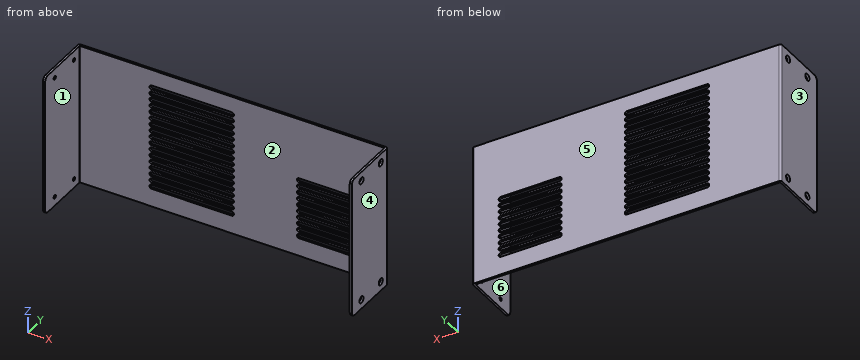
```python
from build123d import *

# Parameters (mm, degrees)
BOSS_EXTRUDE1_DEPTH                             = 132
CSK_FOR_M3_FLAT_HEAD_MACHINE_SCREW1_D           = 3.4
CSK_FOR_M3_FLAT_HEAD_MACHINE_SCREW1_DEPTH       = 5
CSK_FOR_M3_FLAT_HEAD_MACHINE_SCREW1_CSINK_D     = 6.3
CSK_FOR_M3_FLAT_HEAD_MACHINE_SCREW1_CSINK_ANGLE = 90
CSK_FOR_M3_FLAT_HEAD_MACHINE_SCREW1_TIP         = 1.021463052
CSK_FOR_M3_FLAT_HEAD_MACHINE_SCREW2_D           = 3.4
CSK_FOR_M3_FLAT_HEAD_MACHINE_SCREW2_DEPTH       = 5
CSK_FOR_M3_FLAT_HEAD_MACHINE_SCREW2_CSINK_D     = 6.3
CSK_FOR_M3_FLAT_HEAD_MACHINE_SCREW2_CSINK_ANGLE = 90
CSK_FOR_M3_FLAT_HEAD_MACHINE_SCREW2_TIP         = 1.021463052
CUT_EXTRUDE1_DEPTH                              = 5
LPATTERN1_COUNT                                 = 17
LPATTERN1_PITCH                                 = 6
CUT_EXTRUDE2_DEPTH                              = 200
LPATTERN2_COUNT                                 = 10
LPATTERN2_PITCH                                 = 6
FILLET1_R                                       = 4


with BuildPart() as part:
    # Sketch1 → Boss-Extrude1 (new body)
    with BuildSketch(Plane.XY):
        with BuildLine():
            Line((0, 0), (-2, 0))
            Line((-2, 0), (-2, 54.2))
            ThreePointArc((-2, 54.2), (-1.472792206, 55.472792206), (-0.2, 56))
            Line((-0.2, 56), (285.2, 56))
            ThreePointArc((285.2, 56), (286.472792206, 55.472792206), (287, 54.2))
            Line((287, 54.2), (287, 0))
            Line((287, 0), (285, 0))
            Line((285, 0), (285, 53.5))
            ThreePointArc((285, 53.5), (284.853553391, 53.853553391), (284.5, 54))
            Line((284.5, 54), (0.5, 54))
            ThreePointArc((0.5, 54), (0.146446609, 53.853553391), (0, 53.5))
            Line((0, 53.5), (0, 0))
        make_face()
    extrude(amount=BOSS_EXTRUDE1_DEPTH)

    # CSK for M3 Flat Head Machine Screw1
    with Locations(Plane.ZY.offset(2)):
        with Locations((8.5, 45), (8.5, 15), (123.5, 45), (123.5, 15)):
            CounterSinkHole(CSK_FOR_M3_FLAT_HEAD_MACHINE_SCREW1_D / 2, CSK_FOR_M3_FLAT_HEAD_MACHINE_SCREW1_CSINK_D / 2, depth=CSK_FOR_M3_FLAT_HEAD_MACHINE_SCREW1_DEPTH, counter_sink_angle=CSK_FOR_M3_FLAT_HEAD_MACHINE_SCREW1_CSINK_ANGLE)
            with Locations((0, 0, -(CSK_FOR_M3_FLAT_HEAD_MACHINE_SCREW1_DEPTH + CSK_FOR_M3_FLAT_HEAD_MACHINE_SCREW1_TIP / 2))):  # 118° drill point
                Cone(0, CSK_FOR_M3_FLAT_HEAD_MACHINE_SCREW1_D / 2, CSK_FOR_M3_FLAT_HEAD_MACHINE_SCREW1_TIP, mode=Mode.SUBTRACT)

    # CSK for M3 Flat Head Machine Screw2
    with Locations(Plane(origin=(287, 0, 0), x_dir=(0, 0, -1), z_dir=(1, 0, 0))):
        with Locations((-123.5, 45), (-123.5, 15), (-8.5, 45), (-8.5, 15)):
            CounterSinkHole(CSK_FOR_M3_FLAT_HEAD_MACHINE_SCREW2_D / 2, CSK_FOR_M3_FLAT_HEAD_MACHINE_SCREW2_CSINK_D / 2, depth=CSK_FOR_M3_FLAT_HEAD_MACHINE_SCREW2_DEPTH, counter_sink_angle=CSK_FOR_M3_FLAT_HEAD_MACHINE_SCREW2_CSINK_ANGLE)
            with Locations((0, 0, -(CSK_FOR_M3_FLAT_HEAD_MACHINE_SCREW2_DEPTH + CSK_FOR_M3_FLAT_HEAD_MACHINE_SCREW2_TIP / 2))):  # 118° drill point
                Cone(0, CSK_FOR_M3_FLAT_HEAD_MACHINE_SCREW2_D / 2, CSK_FOR_M3_FLAT_HEAD_MACHINE_SCREW2_TIP, mode=Mode.SUBTRACT)

    # Sketch6 → Cut-Extrude1 (cut)
    with BuildSketch(Plane(origin=(0, 56, 0), x_dir=(1, 0, 0), z_dir=(0, 1, 0))):
        with BuildLine():
            Line((67.2, -17), (142.2, -17))
            ThreePointArc((142.2, -17), (144.2, -19), (142.2, -21))
            Line((142.2, -21), (67.2, -21))
            ThreePointArc((67.2, -21), (65.2, -19), (67.2, -17))
        make_face()
    cut_extrude1 = extrude(amount=-CUT_EXTRUDE1_DEPTH, mode=Mode.SUBTRACT)

    # LPattern1: Cut-Extrude1 ×17
    with Locations(*[(0, 0, i * LPATTERN1_PITCH) for i in range(1, LPATTERN1_COUNT)]):
        add(cut_extrude1, mode=Mode.SUBTRACT)

    # Sketch7 → Cut-Extrude2 (cut)
    with BuildSketch(Plane(origin=(0, 56, 0), x_dir=(1, 0, 0), z_dir=(0, 1, 0))):
        with BuildLine():
            Line((205.2, -17), (260.2, -17))
            ThreePointArc((260.2, -17), (262.2, -19), (260.2, -21))
            Line((260.2, -21), (205.2, -21))
            ThreePointArc((205.2, -21), (203.2, -19), (205.2, -17))
        make_face()
    cut_extrude2 = extrude(amount=-CUT_EXTRUDE2_DEPTH, mode=Mode.SUBTRACT)

    # LPattern2: Cut-Extrude2 ×10
    with Locations(*[(0, 0, i * LPATTERN2_PITCH) for i in range(1, LPATTERN2_COUNT)]):
        add(cut_extrude2, mode=Mode.SUBTRACT)

    # Fillet1
    fillet1_edges = [part.edges().sort_by_distance(p)[0] for p in [
        (-1, 0, 0),
        (286, 0, 0),
        (286, 0, 132),
        (-1, 0, 132),
    ]]
    fillet(fillet1_edges, radius=FILLET1_R)


solid = part.part
```
Geometry: final body of the model. Coordinates: model frame, mm. Face numbers are marked on the shaded views. A direction names the side the tool comes from. Coordinates: 2 decimals unless noted, no trailing zeros. Write each loop counter-clockwise with the first axis right and the second up, starting at its lowest first coordinate (ties: lowest second). Pieces come first, ordered by that corner, then holes. Notation, with made-up numbers: M 5,-20 L 17,-20 A27 ccw 17,17 Z; hole C 87,20 d11. An arc over 180 degrees is marked long. Use CSV: the item, a comma, the result in double quotes. Start each with the question number.
1. Ray query, probe 1 along Y at (x, z) = (285.4, 123.5); probe 2 along Z at (x, y) = (285.45, 15); probe 3 along X at (y, z) = (15, 112.5). Return the intervals inside material, ascending.
2. Cut plane A-A on y = 35. Return the cut outline in (x, z).
3. First-contact query: P1, Ø3, axis at x = 203.5, z = 30, coming from the -Y side; P2, Ø4, axis at y = 15, z = 123.5, coming from the -X side. Flat tips, straight axial feed; report the tip coordinate or a pass-through.
4. Mould query, pull axis X, two halves, no side actions, for the marked faces 1, 2, 3 and 4. Classes: pulls with the +X half, pulls with the -X half, needs draft (parallel to the pull), parting line crosses it, or undercut.
5. Cut plane B-B on x = 80. Count the separate pieces of the cut face and the enclosed holes in it, plus the area to 3 significant figures.
6. Cut plane D-D on x = 16.5. Return the cut outline in (y, z).
7. Reachability of the marked faces 5 and 6 from +Z, -Z, +X, -X, +Y, -Y: full face, straight path, thin tool, end or side. Return the list, or none.
Entries:
1,probe 1,"0 to 13.3, 16.7 to 43.3, 46.7 to 55.99"
1,probe 2,"0 to 6.8, 10.2 to 121.8, 125.2 to 132"
1,probe 3,"-2 to 0, 285 to 287"
2,outline,"M -2,0 L 0,0 L 0,132 L -2,132 Z; M 285,0 L 287,0 L 287,132 L 285,132 Z"
3,P1,"y = 54"
3,P2,"x = -0.85"
4,face 1,"undercut"
4,face 2,"undercut"
4,face 3,"pulls with the -X half"
4,face 4,"pulls with the +X half"
5,separate pieces,"18"
5,enclosed holes,"0"
5,area,"128 mm²"
6,outline,"M 54,0 L 56,0 L 56,132 L 54,132 Z"
7,face 5,"+Z, -Z, +X, -X, +Y"
7,face 6,"+Z, -Z, -Y"
